The listing builds one solid part. Answer for the finished solid, in the listing's coordinates (mm). Face numbers are marked on the shaded views. A direction names the side the tool comes from. Coordinates: 2 decimals unless noted, no trailing zeros. Loops run counter-clockwise (first coordinate to the right, second up) from the corner with the lowest first, then second, coordinate; pieces in that order, holes last. Notation, with made-up numbers: (-11, -8) - (36, -8) arc R19 ccw to (36, 24) - close; hole circle Ø10 at (8.5, 71.5). An arc over 180 degrees is marked (long way). Write each question's results on one line, items separated by ' | '. Start each with the question number.
(1) Find section C-C on y = -317. Determine the outline of the cut face in (x, z).
(2) Consider line 1 (Z direction, x = 157, y = -215); line 2 (Z direction, x = 133, y = -285). Determine where each line is inside the solid, lowest interval first. Write a range as from..to.
(3) For the marked faces 4 and 5, determine the directions among +Z, -Z, +X, -X, +Y, -Y from which every point of the face is accessible in a straight line to the end or side of a thin tool.
(4) Determine the mould class of the marked faces 1, 2 and 3 for opening direction Y: released by +Y, released by -Y, zero draft, split by the parting line, or undercut.
(5) Find section A-A on y = -128.5. Determine the outline of the cut face in (x, z), then the cut area to 3 significant figures.
(6) Find section D-D on x = 226. Determine the outline of the cut face in (y, z).
(7) Find section B-B on x = 271. Determine the outline of the cut face in (y, z).
from build123d import *

# Parameters (mm, degrees)
CROQUIS1_W              = 370
CROQUIS1_H              = 430
SALIENTE_EXTRUIR1_DEPTH = 180
CROQUIS2_W              = 185
CROQUIS2_H              = 300
CORTAR_EXTRUIR1_DEPTH   = 12
CROQUIS3_W              = 60
CROQUIS3_H              = 190
CORTAR_EXTRUIR2_DEPTH   = 1


with BuildPart() as part:
    # Croquis1 → Saliente-Extruir1 (new body)
    with BuildSketch(Plane.XY):
        with Locations((185, -215)):
            Rectangle(CROQUIS1_W, CROQUIS1_H)
    extrude(amount=SALIENTE_EXTRUIR1_DEPTH)

    # Croquis2 → Cortar-Extruir1 (cut)
    with BuildSketch(Plane.XY.offset(180)):
        with Locations((185, -215)):
            Rectangle(CROQUIS2_W, CROQUIS2_H)
    extrude(amount=-CORTAR_EXTRUIR1_DEPTH, mode=Mode.SUBTRACT)

    # Croquis3 → Cortar-Extruir2 (cut)
    with BuildSketch(Plane.XY.offset(168)):
        with Locations((145, -180)):
            Rectangle(CROQUIS3_W, CROQUIS3_H)
        with Locations((225, -180)):
            Rectangle(CROQUIS3_W, CROQUIS3_H)
    extrude(amount=-CORTAR_EXTRUIR2_DEPTH, mode=Mode.SUBTRACT)


solid = part.part
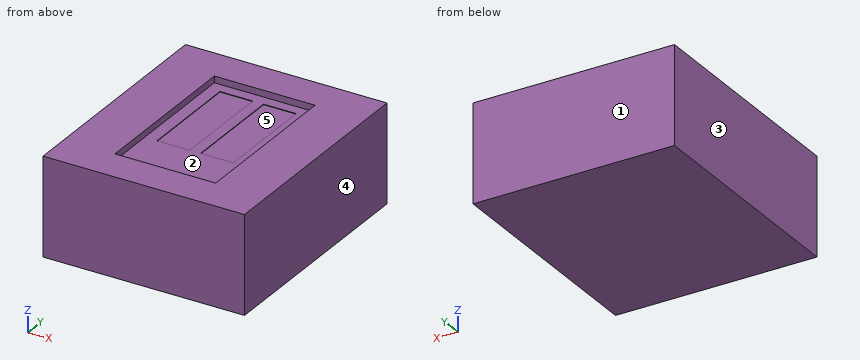
Values:
1) outline: (0, 0) - (370, 0) - (370, 180) - (277.5, 180) - (277.5, 168) - (92.5, 168) - (92.5, 180) - (0, 180) - close
2) line 1: z = 0..167 | line 2: z = 0..168
3) face 4: +Z, -Z, +X, +Y, -Y | face 5: +Z
4) face 1: released by +Y | face 2: undercut | face 3: zero draft
5) outline: (0, 0) - (370, 0) - (370, 180) - (277.5, 180) - (277.5, 168) - (255, 168) - (255, 167) - (195, 167) - (195, 168) - (175, 168) - (175, 167) - (115, 167) - (115, 168) - (92.5, 168) - (92.5, 180) - (0, 180) - close | area: 64,300 mm²
6) outline: (-430, 0) - (0, 0) - (0, 180) - (-65, 180) - (-65, 168) - (-85, 168) - (-85, 167) - (-275, 167) - (-275, 168) - (-365, 168) - (-365, 180) - (-430, 180) - close
7) outline: (-430, 0) - (0, 0) - (0, 180) - (-65, 180) - (-65, 168) - (-365, 168) - (-365, 180) - (-430, 180) - close
